```python
from build123d import *

# Parameters (mm, degrees)
SKETCH1_R           = 135
BOSS_EXTRUDE1_DEPTH = 5
SKETCH2_R           = 132
SKETCH2_R_2         = 127
BOSS_EXTRUDE2_DEPTH = 50


with BuildPart() as part:
    # Sketch1 → Boss-Extrude1 (new, symmetric)
    with BuildSketch(Plane.XY):
        Circle(SKETCH1_R)
    extrude(amount=BOSS_EXTRUDE1_DEPTH, both=True)

    # Sketch2 → Boss-Extrude2 (add)
    with BuildSketch(Plane.XY.offset(5)):
        with Locations(Location((0, 0, 0), (0, 0, 180))):
            Circle(SKETCH2_R)
        with Locations(Location((0, 0, 0), (0, 0, 180))):
            Circle(SKETCH2_R_2, mode=Mode.SUBTRACT)
    extrude(amount=BOSS_EXTRUDE2_DEPTH)


solid = part.part
```
Design review of the part built by this model. Coordinates are the model's own, in mm. A direction names the side the tool comes from. Give positions to 0.01 mm unless a question says otherwise; leave off trailing zeros. Order: outer loops, then holes, each group sorted by start corner. A loop starts at its lowest first (then second) coordinate and runs counter-clockwise, first axis right, second up. Notation, with made-up numbers: (16.25, -16) - (21.25, -16) arc R20 ccw to (21.25, 21) - close; hole circle Ø8 at (14.5, 49.5). An arc over 180 degrees is marked (long way). Use a Markdown table: item, result. Add a question column.
(1) Machinability: for faces 1 (the face through (69, -108, 55)), 2 (the face through (-2, 2, 5)), which of the approach directions +Z, -Z, +X, -X, +Y, -Y give a long, thin tool a straight path to every point of the face, cutting with its end or side? Answer none if there is none.
(2) Clearance check with flat-ended pins moving along their axes: P1, Ø1.5, axis at x = -21.5, z = 31, coming from the -Y side; P2, Ø6, axis at x = -32.5, y = 15.5, coming from the +Z side; P3, Ø3, axis at x = 14, z = 13, coming from the -Y side. State where each tip first meets the part, or that it passes through.
(3) Mouldability with a two-part tool opening along Y and no side actions: class faces 3 (the face through (129, -29, 5)), 4 (the face through (-107.13, -82.15, 0.07)), 5 (the face through (27.53, 123.98, 29.65)) as +Y half, -Y half, draft (parallel to the pull), parting line (faces both ways), or undercut.
(4) Add section A-A on x = 0. Give the boundary of the cut face in (y, z), then the cut area to 3 significant figures.
(5) Add section C-C on z = 17. Give the boundary of the cut face in (x, y), then the cut area to 3 significant figures.
(6) Wall thickness on probe 1 along Y at (x, z) = (0, 34); probe 2 along X at (y, z) = (-49, 46.5); probe 3 along X at (y, z) = (-1.5, 16): over which ranges is each line inside the solid? List them lowest first. Write a range as [from, to].
Report:
| question | item | result |
|---|---|---|
| 1 | face 1 | +Z, +X, -X, +Y, -Y |
| 1 | face 2 | +Z |
| 2 | P1 | stops at y = -130.36 |
| 2 | P2 | stops at z = 5 |
| 2 | P3 | stops at y = -131.41 |
| 3 | face 3 | draft |
| 3 | face 4 | parting line |
| 3 | face 5 | undercut |
| 4 | outline | (-135, -5) - (135, -5) - (135, 5) - (132, 5) - (132, 55) - (127, 55) - (127, 5) - (-127, 5) - (-127, 55) - (-132, 55) - (-132, 5) - (-135, 5) - close |
| 4 | area | 3,200 mm² |
| 5 | outline | circle Ø264 at (0, 0); hole circle Ø254 at (0, 0) |
| 5 | area | 4,070 mm² |
| 6 | probe 1 | y = [-132, -127], [127, 132] |
| 6 | probe 2 | x = [-122.57, -117.17], [117.17, 122.57] |
| 6 | probe 3 | x = [-131.99, -126.99], [126.99, 131.99] |
